CAD build for the part. Positions are in the model's coordinates, mm. A direction names the side the tool comes from. Round coordinates to 2 decimals unless told otherwise and drop trailing zeros. Loops run counter-clockwise (first coordinate to the right, second up) from the corner with the lowest first, then second, coordinate; pieces in that order, holes last. Notation, with made-up numbers: M 20,21.5 L 38,21.5 A11 ccw 38,26.5 Z; hole C 56.25,13 d9. An arc over 180 degrees is marked long. Put each result on its own line as item: value. Start each with the question number.
from build123d import *

# Parameters (mm, degrees)
SKETCH1_W             = 65
SKETCH1_H             = 50
BOSS_EXTRUDE1_DEPTH   = 1.6002
F_2_5MM_DOWEL_HOLE1_D = 2.2
SKETCH4_W             = 18.1
SKETCH4_H             = 15.24
BOSS_EXTRUDE2_DEPTH   = 11.5


with BuildPart() as part:
    # Sketch1 → Boss-Extrude1 (new body)
    with BuildSketch(Plane(origin=(0, 0, 0), x_dir=(1, 0, 0), z_dir=(0, 1, 0))):
        with Locations((32.5, 25)):
            Rectangle(SKETCH1_W, SKETCH1_H)
    extrude(amount=BOSS_EXTRUDE1_DEPTH)

    # Ø2.5mm Dowel Hole1 (through all)
    with Locations(Plane(origin=(0, 1.6002, 0), x_dir=(1, 0, 0), z_dir=(0, 1, 0))):
        with Locations((3, 11.5), (3, 38.5), (27.8, 17), (27.8, 33)):
            Hole(F_2_5MM_DOWEL_HOLE1_D / 2)

    # Sketch4 → Boss-Extrude2 (add)
    with BuildSketch(Plane(origin=(0, 1.6002, 0), x_dir=(1, 0, 0), z_dir=(0, 1, 0))):
        with Locations((62, 41.5)):
            Rectangle(SKETCH4_W, SKETCH4_H)
        with Locations((62, 8.5)):
            Rectangle(SKETCH4_W, SKETCH4_H)
    extrude(amount=BOSS_EXTRUDE2_DEPTH)


solid = part.part
(1) Flat gauge pins, fed straight in: pin 1 Ø3.5 at (x, y) = (59.5, 6) entering from -Z; pin 2 Ø15 at (x, z) = (25.5, -28) entering from +Y; pin 3 Ø6 at (y, z) = (9, -9) entering from -X; pin 4 Ø6.5 at (x, z) = (68, -41) entering from -Y. Where does each tip first touch, or does it go through?
(2) Cut at A-A on z = -11.5. List the corners of the cut face in (x, y), and give its area (3 significant figures).
(3) Mould opens along X. For faces 1 (the cylindrical face through (3.238, 0.789, -10.426)), 2 (the flat face through (71.05, 7, -8)), 3 (the cylindrical face through (27.21, 0.79, -33.93)), 4 (the flat face through (52.95, 7, -8)) say: +X half, -X half, draft (parallel to the pull), parting line (faces both ways), or undercut.
(4) Tool access for faces 5 (the flat face through (68, 1.6, -42)), 6 (the flat face through (62, 7, -0.88)), 7 (the flat face through (62, 7, -33.88)), 8 (the flat face through (32, 1, -50)), 9 (the flat face through (62, 13.1, -42)): list every direction of +Z, -Z, +X, -X, +Y, -Y with a clear straight run to the whole face (end or side of a thin tool).
(5) Cut at C-C on x = 27.8. List the corners of the cut face in (y, z).
(6) Cut at D-D on x = 56. List the corners of the cut face in (y, z), and give its area (3 significant figures).
(7) Cut at B-B on y = 5.75. List the corners of the cut face in (x, z), and give its area (3 significant figures).
(8) Drill centre lines: line 1 along Z through (x, y) = (27.8, 1.2); line 2 along Z through (x, y) = (3, 0.75); line 3 along X through (y, z) = (0.35, -11.5). Where is each one in solid material? Low to high.
Taken from the geometry:
1. pin 1: z = -49.12
1. pin 2: y = 1.6
1. pin 3: x = 52.95
1. pin 4: y = 0
2. outline: M 0,0 L 1.9,0 L 1.9,1.6 L 0,1.6 Z; M 4.1,0 L 65,0 L 65,1.6 L 71.05,1.6 L 71.05,13.1 L 52.95,13.1 L 52.95,1.6 L 4.1,1.6 Z
2. area: 309 mm2
3. face 1: undercut
3. face 2: +X half
3. face 3: undercut
3. face 4: -X half
4. face 5: +Z, -Z, +X, -Y
4. face 6: +Z, +X, -X, +Y
4. face 7: +X, -X, +Y
4. face 8: -Z, +X, -X, +Y, -Y
4. face 9: +Z, -Z, +X, -X, +Y
5. outline: M 0,-50 L 1.6,-50 L 1.6,-34.1 L 0,-34.1 Z; M 0,-31.9 L 1.6,-31.9 L 1.6,-18.1 L 0,-18.1 Z; M 0,-15.9 L 1.6,-15.9 L 1.6,0 L 0,0 Z
6. outline: M 0,-50 L 1.6,-50 L 1.6,-49.12 L 13.1,-49.12 L 13.1,-33.88 L 1.6,-33.88 L 1.6,-16.12 L 13.1,-16.12 L 13.1,-0.88 L 1.6,-0.88 L 1.6,0 L 0,0 Z
6. area: 431 mm2
7. outline: M 52.95,-49.12 L 71.05,-49.12 L 71.05,-33.88 L 52.95,-33.88 Z; M 52.95,-16.12 L 71.05,-16.12 L 71.05,-0.88 L 52.95,-0.88 Z
7. area: 552 mm2
8. line 1: -50 to -34.1, -31.9 to -18.1, -15.9 to 0
8. line 2: -50 to -39.6, -37.4 to -12.6, -10.4 to 0
8. line 3: 0 to 1.9, 4.1 to 65
